The listing builds one solid part. Answer for the finished solid, in the listing's coordinates (mm). A direction names the side the tool comes from. Give positions to 0.01 mm unless a question says otherwise; leave off trailing zeros. Write each loop counter-clockwise with the first axis right and the second up, starting at its lowest first coordinate (ties: lowest second). Pieces come first, ordered by that corner, then holes. Notation, with made-up numbers: (42.25, -1.5) - (68.25, -1.5) arc R23 cw to (68.25, 16.5) - close; hole circle Ø4 at (67, 0). An arc over 180 degrees is marked (long way). Return JSON: item names as keys, results as strings.
from build123d import *

# Parameters (mm, degrees)
EXTRUDE1_DEPTH = 15


with BuildPart() as part:
    # Sketch1 → Extrude1 (new body)
    with BuildSketch(Plane.XY.offset(15)):
        with BuildLine():
            Line((-14.551292676, 3.97958199), (-14.551292676, 4.079606381))
            ThreePointArc((-14.551292676, 4.079606381), (-14.476897799, 4.259211503), (-14.297292676, 4.333606381))
            Line((-14.297292676, 4.333606381), (-12.393373616, 4.333606381))
            ThreePointArc((-12.393373616, 4.333606381), (-12.213768494, 4.259211503), (-12.139373616, 4.079606381))
            Line((-12.139373616, 4.079606381), (-12.139373616, 3.97958199))
            ThreePointArc((-12.139373616, 3.97958199), (-12.032339909, 3.226505542), (-11.719716097, 2.533074433))
            ThreePointArc((-11.719716097, 2.533074433), (-11.618392315, 2.437817098), (-11.483697969, 2.403206381))
            Line((-11.483697969, 2.403206381), (-10.206978323, 2.403206381))
            ThreePointArc((-10.206978323, 2.403206381), (-10.072283977, 2.437817098), (-9.970960196, 2.533074433))
            ThreePointArc((-9.970960196, 2.533074433), (-9.658336383, 3.226505542), (-9.551302676, 3.97958199))
            Line((-9.551302676, 3.97958199), (-9.551302676, 4.079606381))
            ThreePointArc((-9.551302676, 4.079606381), (-9.476907799, 4.259211503), (-9.297302676, 4.333606381))
            Line((-9.297302676, 4.333606381), (-7.393383616, 4.333606381))
            ThreePointArc((-7.393383616, 4.333606381), (-7.213778494, 4.259211503), (-7.139383616, 4.079606381))
            Line((-7.139383616, 4.079606381), (-7.139383616, 3.97958199))
            ThreePointArc((-7.139383616, 3.97958199), (-7.032349909, 3.226505542), (-6.719726097, 2.533074433))
            ThreePointArc((-6.719726097, 2.533074433), (-6.618402315, 2.437817098), (-6.483707969, 2.403206381))
            Line((-6.483707969, 2.403206381), (-5.206988323, 2.403206381))
            ThreePointArc((-5.206988323, 2.403206381), (-5.072293977, 2.437817098), (-4.970970196, 2.533074433))
            ThreePointArc((-4.970970196, 2.533074433), (-4.658346383, 3.226505542), (-4.551312676, 3.97958199))
            Line((-4.551312676, 3.97958199), (-4.551312676, 4.079606381))
            ThreePointArc((-4.551312676, 4.079606381), (-4.476917799, 4.259211503), (-4.297312676, 4.333606381))
            Line((-4.297312676, 4.333606381), (-2.393393616, 4.333606381))
            ThreePointArc((-2.393393616, 4.333606381), (-2.213788494, 4.259211503), (-2.139393616, 4.079606381))
            Line((-2.139393616, 4.079606381), (-2.139393616, 3.97958199))
            ThreePointArc((-2.139393616, 3.97958199), (-2.032359909, 3.226505542), (-1.719736097, 2.533074433))
            ThreePointArc((-1.719736097, 2.533074433), (-1.618412315, 2.437817098), (-1.483717969, 2.403206381))
            Line((-1.483717969, 2.403206381), (-0.206998323, 2.403206381))
            ThreePointArc((-0.206998323, 2.403206381), (-0.072303977, 2.437817098), (0.029019804, 2.533074433))
            ThreePointArc((0.029019804, 2.533074433), (0.341643617, 3.226505542), (0.448677324, 3.97958199))
            Line((0.448677324, 3.97958199), (0.448677324, 4.079606381))
            ThreePointArc((0.448677324, 4.079606381), (0.523072201, 4.259211503), (0.702677324, 4.333606381))
            Line((0.702677324, 4.333606381), (2.606596384, 4.333606381))
            ThreePointArc((2.606596384, 4.333606381), (2.786201506, 4.259211503), (2.860596384, 4.079606381))
            Line((2.860596384, 4.079606381), (2.860596384, 3.97958199))
            ThreePointArc((2.860596384, 3.97958199), (2.967630091, 3.226505542), (3.280253903, 2.533074433))
            ThreePointArc((3.280253903, 2.533074433), (3.381577685, 2.437817098), (3.516272031, 2.403206381))
            Line((3.516272031, 2.403206381), (4.792991677, 2.403206381))
            ThreePointArc((4.792991677, 2.403206381), (4.927686023, 2.437817098), (5.029009804, 2.533074433))
            ThreePointArc((5.029009804, 2.533074433), (5.341633617, 3.226505542), (5.448667324, 3.97958199))
            Line((5.448667324, 3.97958199), (5.448667324, 4.079606381))
            ThreePointArc((5.448667324, 4.079606381), (5.523062201, 4.259211503), (5.702667324, 4.333606381))
            Line((5.702667324, 4.333606381), (6.654626854, 4.333606381))
            Line((6.654626854, 4.333606381), (6.654626854, 6.213206381))
            Line((6.654626854, 6.213206381), (-18.345323146, 6.213206381))
            Line((-18.345323146, 6.213206381), (-18.345323146, 4.333606381))
            Line((-18.345323146, 4.333606381), (-17.393363616, 4.333606381))
            ThreePointArc((-17.393363616, 4.333606381), (-17.213758494, 4.259211503), (-17.139363616, 4.079606381))
            Line((-17.139363616, 4.079606381), (-17.139363616, 3.97958199))
            ThreePointArc((-17.139363616, 3.97958199), (-17.032329909, 3.226505542), (-16.719706097, 2.533074433))
            ThreePointArc((-16.719706097, 2.533074433), (-16.618382315, 2.437817098), (-16.483687969, 2.403206381))
            Line((-16.483687969, 2.403206381), (-15.206968323, 2.403206381))
            ThreePointArc((-15.206968323, 2.403206381), (-15.072273977, 2.437817098), (-14.970950196, 2.533074433))
            ThreePointArc((-14.970950196, 2.533074433), (-14.658326383, 3.226505542), (-14.551292676, 3.97958199))
        make_face()
    extrude(amount=-EXTRUDE1_DEPTH)


solid = part.part
Item 1: A flat-ended cylindrical pin translates along its axis: P1, Ø1, axis at x = -18, z = 7.5, coming from the -Y side. Find the tip coordinate at first contact, or state that the pin passes through.
Answer below:
{"P1": "stops at y = 4.33"}
Item 2: The mould has two halves that part along X. Classify faces 1 (the face through (6.655, 5, 8)), 2 (the face through (4, 2.403, 8)), 3 (the face through (-12.035, 3.237, 7.605)): +X half, -X half, draft (parallel to the pull), parting line (faces both ways), or undercut.
Answer below:
{"face 1": "+X half", "face 2": "draft", "face 3": "undercut"}
Item 3: A cutting plane is placed at B-B on x = -2.75. Determine the outline of the cut face in (y, z).
Answer below:
{"outline": "(4.33, 0) - (6.21, 0) - (6.21, 15) - (4.33, 15) - close"}
Item 4: A cutting plane is placed at A-A on y = 3.65. Determine the outline of the cut face in (x, z).
Answer below:
{"outline": "(-17.12, 0) - (-14.57, 0) - (-14.57, 15) - (-17.12, 15) - close; (-12.12, 0) - (-9.57, 0) - (-9.57, 15) - (-12.12, 15) - close; (-7.12, 0) - (-4.57, 0) - (-4.57, 15) - (-7.12, 15) - close; (-2.12, 0) - (0.43, 0) - (0.43, 15) - (-2.12, 15) - close; (2.88, 0) - (5.43, 0) - (5.43, 15) - (2.88, 15) - close"}
Item 5: Consider L1, parallel to X at y = 4.05, z = 4; L2, parallel to X at y = 4.25, z = 6.25 (3 decimals); L3, parallel to Y at x = 2.5, z = 9.5. Determine where each line is inside the solid, lowest interval first.
Answer below:
{"L1": "x = -17.14 to -14.55, -12.14 to -9.55, -7.14 to -4.55, -2.14 to 0.45, 2.86 to 5.45", "L2": "x = -17.205 to -14.486, -12.205 to -9.486, -7.205 to -4.486, -2.205 to 0.514, 2.795 to 5.514", "L3": "y = 4.33 to 6.21"}
Item 6: For faces 4 (the face through (-14.66, 3.22, 7.6)), 5 (the face through (-17.035, 3.237, 7.605)), determine the directions among +Z, -Z, +X, -X, +Y, -Y from which every point of the face is accessible in a straight line to the end or side of a thin tool.
Answer below:
{"face 4": "+Z, -Z, -Y", "face 5": "+Z, -Z, -X, -Y"}
